Geometry: final body of the model. Coordinates: model frame, mm. A direction names the side the tool comes from. Give positions to 0.01 mm unless a question says otherwise; leave off trailing zeros. Loops run counter-clockwise (first coordinate to the right, second up) from the corner with the lowest first, then second, coordinate; pieces in that order, holes last. Notation, with made-up numbers: (37.5, 82.25) - (84.5, 82.25) arc R35 ccw to (84.5, 121.25) - close; hole circle Ø7 at (41.5, 4.25). An arc over 180 degrees is marked (long way). Use one line per item in the form item = value.
Solid Edge part; units mm, degrees
sketch "Sketch1" plane through (0, 0, 0) normal (0, 0, 1) x (1, 0, 0)
  circle A0 centre (0, 0) radius 14
extrude "Protrusion1" add sketch "Sketch1" along normal blind 19
sketch "Sketch2" plane through (0, 0, 19) normal (0, 0, 1) x (1, 0, 0)
  line L0 (-17.5, -3.5) -> (-13.5554, -3.5)
  arc A0 (-13.5554, -3.5) -> (-13.5554, 3.5) centre (0, 0) cw
  line L1 (-17.5, 3.5) -> (-13.5554, 3.5)
  arc A1 (-17.5, -3.5) -> (-17.5, 3.5) centre (-17.5, 0) cw
  circle A2 centre (-17.5, 0) radius 2.1
  circle A3 centre (17.5, 0) radius 2.1
  line L2 (17.5, -3.5) -> (13.5554, -3.5)
  line L3 (17.5, 3.5) -> (13.5554, 3.5)
  arc A4 (17.5, 3.5) -> (17.5, -3.5) centre (17.5, 0) cw
  arc A5 (13.5554, 3.5) -> (13.5554, -3.5) centre (0, 0) cw
extrude "ExtrudedProtrusion_2" add sketch "Sketch2" against normal blind 0.7
sketch "Sketch3" plane through (0, 0, 19) normal (0, 0, 1) x (1, 0, 0)
  circle A0 centre (0, 8) radius 4.5
extrude "ExtrudedProtrusion_3" add sketch "Sketch3" along normal blind 1.5
sketch "Sketch4" plane through (0, 8, 20.5) normal (0, 0, 1) x (1, 0, 0)
  circle A0 centre (0, 0) radius 2.5
extrude "ExtrudedProtrusion_4" add sketch "Sketch4" along normal blind 2.5
sketch "Sketch5" plane through (0, 8, 23) normal (0, 0, 1) x (1, 0, 0)
  line L0 (-1.5, 2) -> (-1.5, -2)
  line L1 (1.5, 2) -> (1.5, -2)
  arc A0 (-1.5, 2) -> (1.5, 2) centre (0, 0) cw
  arc A1 (1.5, -2) -> (-1.5, -2) centre (0, 0) cw
extrude "ExtrudedProtrusion_5" add sketch "Sketch5" along normal blind 6
sketch "Sketch6" plane through (0, 0, 19) normal (0, 0, 1) x (1, 0, 0)
  line L0 (-7.3, -17) -> (7.3, -17)
  line L1 (7.3, -17) -> (7.3, -11.9461)
  line L2 (-7.3, -17) -> (-7.3, -11.9461)
  arc A0 (7.3, -11.9461) -> (-7.3, -11.9461) centre (0, 0) cw
extrude "Protrusion2" add sketch "Sketch6" against normal up to vertex (19 mm away)
(1) Material intervals for L1, parallel to Y at x = -17.5, z = 18.85; L2, parallel to Z at x = -5.5, y = -6.5; L3, parallel to Z at x = 0, y = 11.5, sorted ascending. Write a range as from..to.
Solution:
L1 = -3.5..-2.1, 2.1..3.5
L2 = 0..19
L3 = 0..20.5
(2) Pull-direction query (Y, two-part tool) for faces 1 (the face through (19.503, 0.631, 18.655)), 2 (the face through (0, 8, 29)), 3 (the face through (-15.497, 0.631, 18.655)), 4 (the face through (1.15, 10.22, 23.75)); classes: released by +Y, released by -Y, zero draft, split by the parting line, or undercut.
Solution:
face_1 = undercut
face_2 = zero draft
face_3 = undercut
face_4 = split by the parting line
(3) Cut plane B-B (x = 0). Return the cut outline in (y, z), plus the area to 3 significant figures.
Solution:
outline = (-17, 0) - (14, 0) - (14, 19) - (12.5, 19) - (12.5, 20.5) - (10.5, 20.5) - (10.5, 29) - (5.5, 29) - (5.5, 20.5) - (3.5, 20.5) - (3.5, 19) - (-17, 19) - close
area = 645 mm2
(4) Cut plane C-C (y = 11.5). Return the cut outline in (x, z), plus the area to 3 significant figures.
Solution:
outline = (-7.98, 0) - (7.98, 0) - (7.98, 19) - (2.83, 19) - (2.83, 20.5) - (-2.83, 20.5) - (-2.83, 19) - (-7.98, 19) - close
area = 312 mm2
(5) Pin query (flat end, axial travel): P1, Ø0.8, axis at x = 15.5, z = 18.5, coming from the +Y side; P2, Ø0.8, axis at x = 2, y = 8.5, coming from the +Z side; P3, Ø1.2, axis at y = 8, z = 27.5, coming from the +X side. Return the tip coordinate at first contact, or that it passes through.
Solution:
P1 = 3.5
P2 = 23
P3 = 1.5
(6) Cut plane A-A (y = 0). Return the cut outline in (x, z).
Solution:
outline = (-21, 18.3) - (-19.6, 18.3) - (-19.6, 19) - (-21, 19) - close; (-15.4, 18.3) - (-14, 18.3) - (-14, 0) - (14, 0) - (14, 18.3) - (15.4, 18.3) - (15.4, 19) - (-15.4, 19) - close; (19.6, 18.3) - (21, 18.3) - (21, 19) - (19.6, 19) - close
(7) Cut plane D-D (z = 7.75). Return the cut outline in (x, y).
Solution:
outline = (-7.3, -17) - (7.3, -17) - (7.3, -11.95) arc R14 ccw (long way) to (-7.3, -11.95) - close
(8) Access query for faces 5 (the face through (-0.51, 13.99, 9.37)), 6 (the face through (1.5, 8, 26)), 7 (the face through (-0.98, 12.39, 19.74)). Directions: +Z, -Z, +X, -X, +Y, -Y. A direction counts if a zero-diameter tool reaches every point of the face in a straight line with its end or side. Return the directions, or none.
Solution:
face_5 = -Z
face_6 = +Z, +X, +Y, -Y
face_7 = +Z
